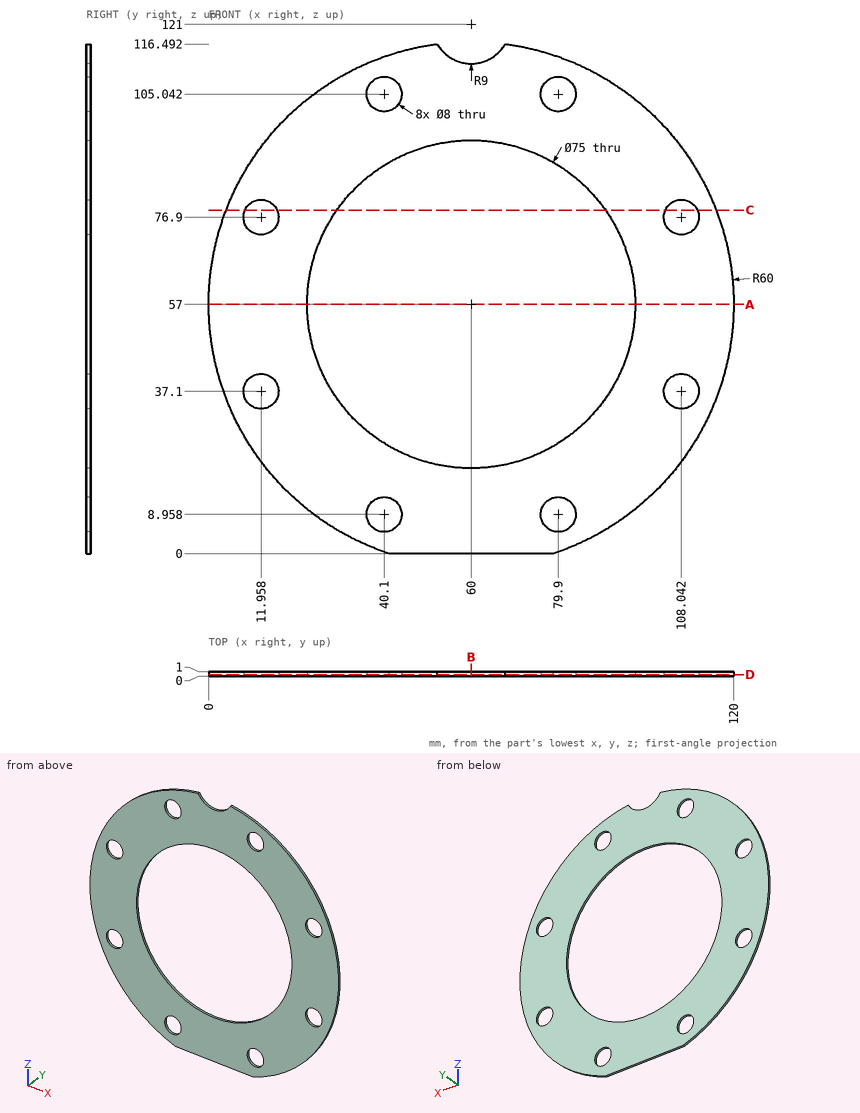
The figure shows three views and two pictorial views of one solid part (mm, origin at its lowest corner). Answer the questions. Give positions to 0.01 mm unless a question says otherwise; leave off trailing zeros. Order: outer loops, then holes, each group sorted by start corner. A loop starts at its lowest first (then second) coordinate and runs counter-clockwise, first axis right, second up. Notation, with made-up numbers: (-7, 59) - (38, 59) arc R17 ccw to (38, 88) - close; hole circle Ø10 at (10.25, 37). An arc over 180 degrees is marked (long way). Answer as CSV lines item,"result".
Q1. A cutting plane is placed at D-D, the plane y = 0.3. Count the separate pieces of the cut face and the enclosed holes in it, and give its area (3 significant figures).
Answer key:
separate pieces,"1"
enclosed holes,"9"
area,"6,360 mm^2"
Q2. Straight lines are drawn through the part: L1, parallel to X at y = 0.4, z = 57; L2, parallel to Z at x = 82.5, y = 0.9; L3, parallel to Z at x = 88, y = 0.2 (1 decimal). For each, find the intervals that lie inside material, in ascending order.
Answer key:
L1,"x = 0 to 22.5, 97.5 to 120"
L2,"z = 1.38 to 5.92, 12 to 27, 87 to 102, 108.08 to 112.62"
L3,"z = 3.9 to 32.1, 81.9 to 110.1"
Q3. A cutting plane is placed at C-C, the plane z = 78.5. Determine the outline of the cut face in (x, y) (1 decimal).
Answer key:
outline,"(4, 0) - (8.3, 0) - (8.3, 1) - (4, 1) - close; (15.6, 0) - (29.3, 0) - (29.3, 1) - (15.6, 1) - close; (90.7, 0) - (104.4, 0) - (104.4, 1) - (90.7, 1) - close; (111.7, 0) - (116, 0) - (116, 1) - (111.7, 1) - close"
Q4. A cutting plane is placed at B-B, the plane x = 60. Determine the outline of the cut face in (y, z).
Answer key:
outline,"(0, 0) - (1, 0) - (1, 19.5) - (0, 19.5) - close; (0, 94.5) - (1, 94.5) - (1, 112) - (0, 112) - close"
Q5. This flat-tipped pin is pushed along its axis until it touches: pin 1 Ø7 at (x, z) = (79.9, 8.96) entering from -Y. Where does it stop, or does it pass through?
Answer key:
pin 1,"passes through"
Q6. A cutting plane is placed at A-A, the plane z = 57. Determine the outline of the cut face in (x, y).
Answer key:
outline,"(0, 0) - (22.5, 0) - (22.5, 1) - (0, 1) - close; (97.5, 0) - (120, 0) - (120, 1) - (97.5, 1) - close"
